Read the model definition and answer for the solid it produces. Units are mm, in the model's axes. Face numbers are marked on the shaded views. A direction names the side the tool comes from. Round coordinates to 2 decimals unless told otherwise and drop trailing zeros. Order: outer loops, then holes, each group sorted by start corner. A loop starts at its lowest first (then second) coordinate and runs counter-clockwise, first axis right, second up. Notation, with made-up numbers: (71, -31) - (116, -31) arc R29 ccw to (116, -6) - close; hole circle Ø6 at (74, -26). An arc over 180 degrees is marked (long way). Put each result on its own line as item: value. Start each with the question number.
Q1. For a pull along X with two mould halves and no side action, classify the marked faces 1, 2 and 3 as pulls with the +X half, pulls with the -X half, needs draft (parallel to the pull), parting line crosses it, or undercut.
Q2. Section D-D on x = 13 is taken. Give the vertices of the cut face in (y, z), then the cut area to 3 significant figures.
Q3. Which of the six approach directions +Z, -Z, +X, -X, +Y, -Y give full straight-line access (tool end or side, diameter ignored) to the marked faces 4, 5 and 6?
Q4. Section B-B on z = 0.85 is taken. Give the vertices of the cut face in (x, y), then the cut area to 3 significant figures.
Q5. Find the intervals of material crossed by line 1 along X through (y, z) = (-0.25, 1.4); line 2 along X through (y, z) = (8.5, 1.15); line 3 along Y through (x, z) = (44, 3.2), in increasing order. Write a range as from..to.
Q6. Section C-C on y = 12.75 is taken. Give the vertices of the cut face in (x, z).
Q7. Each of these flat-tipped pins is pushed along its axis until it touches: pin 1 Ø1.2 at (y, z) = (9, 3) entering from +X; pin 2 Ø2 at (y, z) = (10.5, 3) entering from -X; pin 3 Ø2 at (y, z) = (-2, 4.5) entering from +X. Where does it stop, or does it pass through?
Q8. Section A-A on y = -1 is taken. Give the vertices of the cut face in (x, z), then the cut area to 3 significant figures.
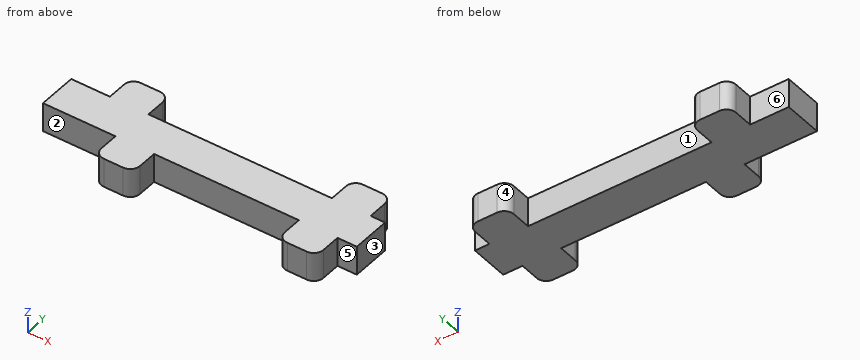
Autodesk Inventor part; units mm, degrees
ref_plane "YZ Plane" through (0, 0, 0) normal (1, 0, 0) x (0, 1, 0)
ref_plane "XZ Plane" through (0, 0, 0) normal (0, 1, 0) x (-1, 0, 0)
ref_plane "XY Plane" through (0, 0, 0) normal (0, 0, 1) x (1, 0, 0)
sketch "Sketch1" plane through (0, 0, 0) normal (0, 0, 1) x (1, 0, 0)
  line L0 (0, 0) -> (65, 0)
  line L1 (65, 0) -> (65, 8)
  line L2 (65, 8) -> (0, 8)
  line L3 (0, 8) -> (0, 0)
  dimension "d0" = 8
  dimension "d1" = 65
extrude "Extrusion1" add sketch "Sketch1" along normal blind 6
sketch "Sketch2" plane through (0, 0, 6) normal (0, 0, 1) x (1, 0, 0)
  line L0 (0, 0) -> (65, 0)
  line L1 (65, 8) -> (0, 8)
  line L2 (0, 8) -> (0, 0)
  line L3 (15, 0) -> (23, 0)
  line L4 (23, 0) -> (23, -4)
  line L5 (21, -6) -> (17, -6)
  line L6 (15, -4) -> (15, 0)
  line L7 (53, 0) -> (61, 0)
  line L8 (61, 0) -> (61, -4)
  line L9 (59, -6) -> (55, -6)
  line L10 (53, -4) -> (53, 0)
  line L11 (8, 8) -> (16, 8)
  line L12 (16, 8) -> (16, 12)
  line L13 (14, 14) -> (10, 14)
  line L14 (8, 12) -> (8, 8)
  line L15 (54, 8) -> (62, 8)
  line L16 (62, 8) -> (62, 12)
  line L17 (60, 14) -> (56, 14)
  line L18 (54, 12) -> (54, 8)
  arc A0 (15, -4) -> (17, -6) centre (17, -4) ccw
  arc A1 (21, -6) -> (23, -4) centre (21, -4) ccw
  arc A2 (10, 14) -> (8, 12) centre (10, 12) ccw
  arc A3 (16, 12) -> (14, 14) centre (14, 12) ccw
  arc A4 (56, 14) -> (54, 12) centre (56, 12) ccw
  arc A5 (62, 12) -> (60, 14) centre (60, 12) ccw
  arc A6 (53, -4) -> (55, -6) centre (55, -4) ccw
  arc A7 (59, -6) -> (61, -4) centre (59, -4) ccw
  dimension "d4" = 2
  dimension "d5" = 8
  dimension "d6" = 6
  dimension "d7" = 6
  dimension "d8" = 8
  dimension "d9" = 8
  dimension "d10" = 8
  dimension "d11" = 15
  dimension "d12" = 30
  dimension "d13" = 8
  dimension "d14" = 38
extrude "Extrusion2" add sketch "Sketch2" against normal blind 6
properties part number "x_motor_smooth_rod_spacer"
Findings:
1. face 1: undercut
1. face 2: needs draft
1. face 3: pulls with the +X half
2. outline: (0, 0) - (14, 0) - (14, 6) - (0, 6) - close
2. area: 84.0 mm2
3. face 4: +Z, -Z, +Y
3. face 5: +Z, -Z, +X, -Y
3. face 6: +Z, -Z, -X, +Y
4. outline: (0, 0) - (15, 0) - (15, -4) arc R2 ccw to (17, -6) - (21, -6) arc R2 ccw to (23, -4) - (23, 0) - (53, 0) - (53, -4) arc R2 ccw to (55, -6) - (59, -6) arc R2 ccw to (61, -4) - (61, 0) - (65, 0) - (65, 8) - (62, 8) - (62, 12) arc R2 ccw to (60, 14) - (56, 14) arc R2 ccw to (54, 12) - (54, 8) - (16, 8) - (16, 12) arc R2 ccw to (14, 14) - (10, 14) arc R2 ccw to (8, 12) - (8, 8) - (0, 8) - close
4. area: 705 mm2
5. line 1: 15..23, 53..61
5. line 2: 8..16, 54..62
5. line 3: 0..8
6. outline: (8.15, 0) - (15.85, 0) - (15.85, 6) - (8.15, 6) - close; (54.15, 0) - (61.85, 0) - (61.85, 6) - (54.15, 6) - close
7. pin 1: x = 62
7. pin 2: x = 8
7. pin 3: x = 61
8. outline: (15, 0) - (23, 0) - (23, 6) - (15, 6) - close; (53, 0) - (61, 0) - (61, 6) - (53, 6) - close
8. area: 96.0 mm2
